Source: CAD feature listing. Evaluate the final solid. Frame: model axes, mm. A direction names the side the tool comes from. Coordinates: 2 decimals unless noted, no trailing zeros. Order: outer loops, then holes, each group sorted by start corner. A loop starts at its lowest first (then second) coordinate and runs counter-clockwise, first axis right, second up.
```python
from build123d import *

# Parameters (mm, degrees)
BOSS_EXTRUDE1_DEPTH     = 3.175
CUT_EXTRUDE1_DEPTH      = 65.189801711
CUT_EXTRUDE1_DEPTH_BACK = 65.189801711
SKETCH3_R               = 1.0922
SKETCH3_R_2             = 1.35
SKETCH3_R_3             = 1.7
SKETCH3_W               = 7
SKETCH3_H               = 15
SKETCH5_W               = 6
SKETCH5_H               = 4.4
CUT_EXTRUDE2_DEPTH      = 65.189801711


with BuildPart() as part:
    # Sketch2 → Boss-Extrude1 (new body)
    with BuildSketch(Plane(origin=(0, 0, 0), x_dir=(1, 0, 0), z_dir=(0, 1, 0))):
        with BuildLine():
            Line((48, 42.5), (-48, 42.5))
            Line((-48, 42.5), (-48, -10.75))
            add(Edge.make_bspline(
                [(-48, -10.75), (-48, -53.083333333), (48, -53.083333333), (48, -10.75)],
                knots=[0, 0, 0, 0, 1, 1, 1, 1], degree=3))
            Line((48, -10.75), (48, 42.5))
        make_face()
    extrude(amount=BOSS_EXTRUDE1_DEPTH)

    # Sketch3 → Cut-Extrude1 (cut, two sides: drawn at the far end of the back side and taken through both)
    with BuildSketch(Plane(origin=(0, 3.175, 0), x_dir=(1, 0, 0), z_dir=(0, 1, 0)).offset(-CUT_EXTRUDE1_DEPTH_BACK)):
        with Locations(Location((-41.5, 36, 0), (0, 0, 270))):
            Circle(SKETCH3_R)
        with Locations(Location((-41.5, 18, 0), (0, 0, 270))):
            Circle(SKETCH3_R)
        with Locations(Location((-30, 19, 0), (0, 0, 270))):
            Circle(SKETCH3_R_2)
        with Locations(Location((41.5, 18, 0), (0, 0, 90))):
            Circle(SKETCH3_R)
        with Locations(Location((41.5, 36, 0), (0, 0, 90))):
            Circle(SKETCH3_R)
        with Locations(Location((-30, -26, 0), (0, 0, 270))):
            Circle(SKETCH3_R_2)
        with Locations(Location((30, -26, 0), (0, 0, 90))):
            Circle(SKETCH3_R_2)
        with Locations(Location((30, 19, 0), (0, 0, 90))):
            Circle(SKETCH3_R_2)
        with Locations(Location((-8.225, -37.5, 0), (0, 0, 270))):
            Circle(SKETCH3_R_3)
        with Locations(Location((8.225, -37.5, 0), (0, 0, 90))):
            Circle(SKETCH3_R_3)
        with Locations(Location((0, -23.253882108, 0), (0, 0, 90))):
            Circle(SKETCH3_R_3)
        with Locations((-17.68, 27)):
            Rectangle(SKETCH3_W, SKETCH3_H)
        with Locations((17.68, 27)):
            Rectangle(SKETCH3_W, SKETCH3_H)
    extrude(amount=CUT_EXTRUDE1_DEPTH + CUT_EXTRUDE1_DEPTH_BACK, mode=Mode.SUBTRACT)

    # Sketch5 → Cut-Extrude2 (cut, through all)
    with BuildSketch(Plane(origin=(0, 3.175, 0), x_dir=(1, 0, 0), z_dir=(0, 1, 0))):
        with Locations((24, 40.3)):
            Rectangle(SKETCH5_W, SKETCH5_H)
        with Locations((-24, 40.3)):
            Rectangle(SKETCH5_W, SKETCH5_H)
    extrude(amount=-CUT_EXTRUDE2_DEPTH, mode=Mode.SUBTRACT)


solid = part.part
```
Q1. Set-up query: faces 1 (the flat face through (48, 2, -16)), 2 (the flat face through (27, 2, -40)), 3 (the flat face through (-18, 2, -19.5)). Return all of +Z, -Z, +X, -X, +Y, -Y with unobstructed straight access to the full face (end or side cutting, diameter ignored); none if empty.
Solutions:
face 1: +Z, -Z, +X, +Y, -Y
face 2: -Z, +Y, -Y
face 3: +Y, -Y
Q2. Section query B-B on x = 41.5. Give the number of separate pieces and of enclosed holes in the cut face, plus the area to 3 significant figures.
Solutions:
separate pieces: 3
enclosed holes: 0
area: 209 mm2
Q3. Pull-direction query (X, two-part tool) for faces 4 (the flat face through (-24, 2, -38.1)), 5 (the flat face through (21, 2, -40)), 6 (the flat face through (-37, 2, -42.5)), 7 (the flat face through (-48, 2, -16)); classes: pulls with the +X half, pulls with the -X half, needs draft (parallel to the pull), parting line crosses it, or undercut.
Solutions:
face 4: undercut
face 5: undercut
face 6: needs draft
face 7: pulls with the -X half
Q4. Section query A-A on z = -30.5. Output: boundary loops of the cut face in (x, y) (3 decimals).
Solutions:
outline: (-48, 0) - (-21.18, 0) - (-21.18, 3.175) - (-48, 3.175) - close; (-14.18, 0) - (14.18, 0) - (14.18, 3.175) - (-14.18, 3.175) - close; (21.18, 0) - (48, 0) - (48, 3.175) - (21.18, 3.175) - close
Q5. Pin query (flat end, axial travel): P1, Ø1.7, axis at x = 41.5, z = -18, coming from the +Y side; P2, Ø1, axis at x = -24, y = 1.5, coming from the -Z side. Return the tip coordinate at first contact, or that it passes through.
Solutions:
P1: passes through
P2: stops at z = -38.1
Q6. Material intervals for line 1 along X through (y, z) = (0.7, -30); line 2 along X through (y, z) = (0.75, -36); line 3 along Z through (x, y) = (-42, 1.45), sorted ascending.
Solutions:
line 1: x = -48 to -21.18, -14.18 to 14.18, 21.18 to 48
line 2: x = -48 to -42.59, -40.41 to 40.41, 42.59 to 48
line 3: z = -42.5 to -36.97, -35.03 to -18.97, -17.03 to 27.14
